For this review, take the finished solid that the model builds, in its own axes (mm). A direction names the side the tool comes from. Give positions to 0.01 mm unless a question says otherwise; leave off trailing zeros. Loops run counter-clockwise (first coordinate to the right, second up) from the corner with the lowest first, then second, coordinate; pieces in that order, holes last.
```python
from build123d import *

# Parameters (mm, degrees)
BLANKSKE_W          = 100
BLANKSKE_H          = 11.5
BLANK_DEPTH         = 10
TOOTHCUTSIM_DEPTH   = 102.154584671
TEETHCUTS_COUNT     = 22
TEETHCUTS_PITCH     = 4.712388975
SKETCH2_W           = 40
SKETCH2_H           = 3
SKETCH2_W_2         = 34.0000508
BOSS_EXTRUDE1_DEPTH = 100


with BuildPart() as part:
    # BlankSke → Blank (new body)
    with BuildSketch(Plane.XY):
        with Locations((50, 5.75)):
            Rectangle(BLANKSKE_W, BLANKSKE_H)
    extrude(amount=-BLANK_DEPTH)

    # TooCutSkeSim → ToothCutSim (cut, through all)
    with BuildSketch(Plane.XY):
        Polygon((0.654653055, 8.125), (-0.654653055, 8.125), (-1.892297439, 11.5254), (1.892297439, 11.5254), align=None)
    toothcutsim = extrude(amount=-TOOTHCUTSIM_DEPTH, mode=Mode.SUBTRACT)

    # TeethCuts: ToothCutSim ×22
    with Locations(*[(i * TEETHCUTS_PITCH, 0, 0) for i in range(1, TEETHCUTS_COUNT)]):
        add(toothcutsim, mode=Mode.SUBTRACT)

    # Sketch2 → Boss-Extrude1 (add)
    with BuildSketch(Plane(origin=(100, 0, 0), x_dir=(0, 0, -1), z_dir=(1, 0, 0))):
        with Locations((-20, 1.5)):
            Rectangle(SKETCH2_W, SKETCH2_H)
        with Locations((27.0000254, 1.5)):
            Rectangle(SKETCH2_W_2, SKETCH2_H)
        Polygon((44.0000508, -3), (44.0000508, 0), (10, 0), (0, 0), (-40, 0), (-40, -3), align=None)
    extrude(amount=-BOSS_EXTRUDE1_DEPTH)


solid = part.part
```
Item 1: Clearance check with flat-ended pins moving along their axes: pin 1 Ø1.5 at (x, y) = (12, 10) entering from +Z; pin 2 Ø1 at (x, z) = (47.5, 5.5) entering from +Y; pin 3 Ø0.7 at (x, z) = (37.5, -6) entering from +Y (3 decimals); pin 4 Ø1.5 at (y, z) = (4, 12.5) entering from +X. State where each tip first meets the part, or that it passes through.
Answer:
pin 1: stops at z = 0
pin 2: stops at y = 3
pin 3: stops at y = 8.125
pin 4: passes through
Item 2: The part is to be moulded in two halves that separate along X. For faces 1 (the flat face through (0, 0, -1)), 2 (the flat face through (49, 6, 0)), 3 (the flat face through (15.4, 9.8, -4.9)), say which applies: released by +X, released by -X, zero draft, split by the parting line, or undercut.
Answer:
face 1: released by -X
face 2: zero draft
face 3: undercut
Item 3: Take a section at A-A on z = -17. Give the boundary of the cut face in (x, y).
Answer:
outline: (0, -3) - (100, -3) - (100, 3) - (0, 3) - close
Item 4: For L1, parallel to Y at x = 20.5, z = 1; L2, parallel to Z at x = 35, y = 9.5, list the stretches that pass through material, from the lowest coordinate up.
Answer:
L1: y = -3 to 3
L2: z = -10 to 0
Item 5: Tool access review of faces 4 (the flat face through (88.275, 9.789, -4.93)), 5 (the flat face through (51, -3, -1)), 6 (the flat face through (51, 3, -27)): name each direction out of +Z, -Z, +X, -X, +Y, -Y from which nothing blocks a thin tool from reaching the whole face with its end or side.
Answer:
face 4: +Z, -Z, +Y
face 5: +Z, -Z, +X, -X, -Y
face 6: -Z, +X, -X, +Y
Item 6: Take a section at B-B on y = 4.75. Give the boundary of the cut face in (x, z).
Answer:
outline: (0, -10) - (100, -10) - (100, 0) - (0, 0) - close
